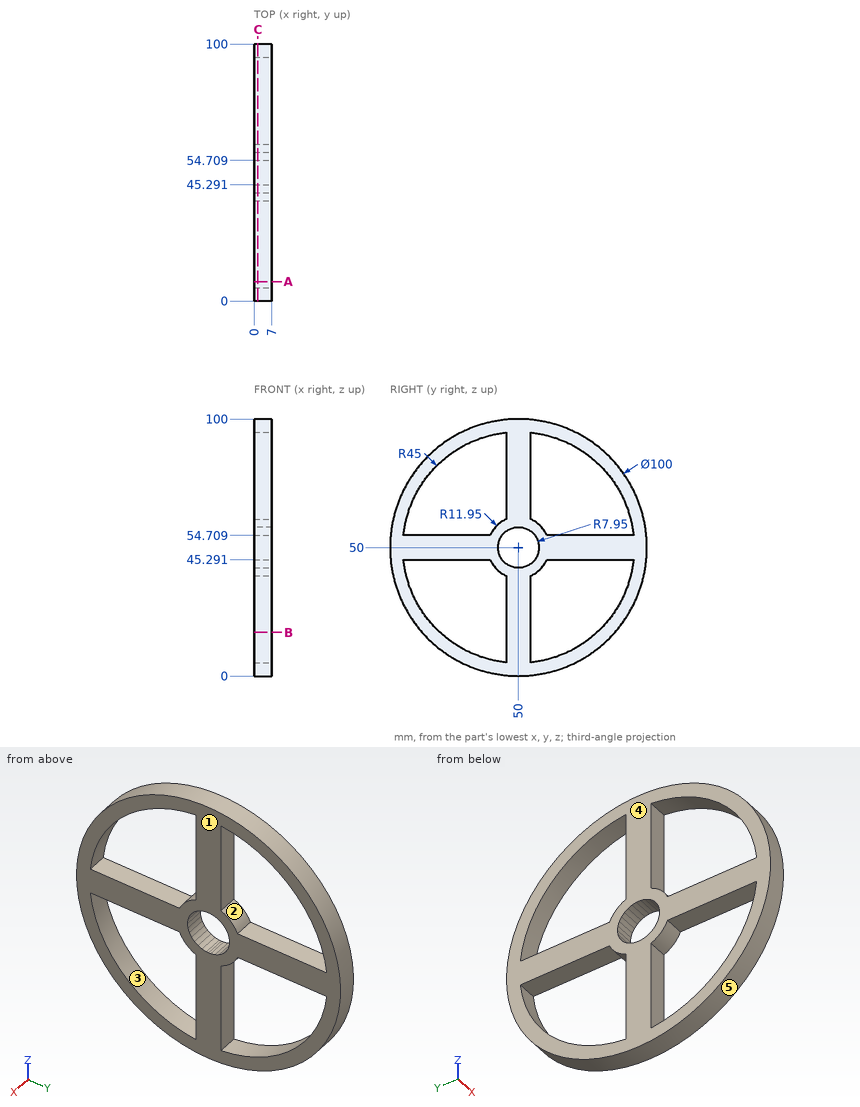
The drawing under review shows one solid part. Ordinate dimensions are in mm from its lowest x, y, z. A direction names the side the tool comes from. Coordinates: 2 decimals unless noted, no trailing zeros. Loops run counter-clockwise (first coordinate to the right, second up) from the corner with the lowest first, then second, coordinate; pieces in that order, holes last.
Item 1: Draft analysis for pull direction Y (two halves, no side actions). For the marked faces 3, 4 and 5, state which applies: pulls with the +Y half, pulls with the -Y half, needs draft (parallel to the pull), parting line crosses it, or undercut.
Completed:
face 3: undercut
face 4: needs draft
face 5: parting line crosses it
Item 2: Clearance check with flat-ended pins moving along their axes: pin 1 (2 mm diameter, centred on x = 4.5, z = 29.5, fed in from +Y); pin 2 (2 mm diameter, centred on x = 4.5, y = 79, fed in from +Z) (1 decimal); pin 3 (2 mm diameter, centred on x = 3, z = 41, fed in from -Y); pin 4 (3 mm diameter, centred on y = 82, z = 42.5, fed in from -X). State where each tip first meets the part, or that it passes through.
Completed:
pin 1: stops at y = 96.04
pin 2: stops at z = 91.4
pin 3: stops at y = 0.64
pin 4: passes through
Item 3: For the marked faces 1 and 2, list the 3-axis set-ups (+Z, -Z, +X, -X, +Y, -Y) from which the entire face can be reached by the end or side of a thin tool; tool diameter is ignored.
Completed:
face 1: +Z, -Z, +X, +Y, -Y
face 2: +X, -X
Item 4: Add section C-C (x = 1.5). Give the number of separate pieces and of enclosed holes in the cut face, and give its area (3 significant figures).
Completed:
separate pieces: 1
enclosed holes: 5
area: 3,000 mm2
Item 5: Add section B-B (z = 17). Write out the cut boundary in (x, y).
Completed:
outline: (0, 12.44) - (7, 12.44) - (7, 19.41) - (0, 19.41) - close; (0, 45.29) - (7, 45.29) - (7, 54.71) - (0, 54.71) - close; (0, 80.59) - (7, 80.59) - (7, 87.56) - (0, 87.56) - close
Item 6: Wall thickness on L1, parallel to Z at x = 5.25, y = 77; L2, parallel to Y at x = 1.75, z = 72.5; L3, parallel to Y at x = 4.5, z = 41: over which ranges is each line inside the solid? List them lowest first.
Completed:
L1: z = 7.92 to 14, 45.29 to 54.71, 86 to 92.08
L2: y = 5.35 to 11.03, 45.29 to 54.71, 88.97 to 94.65
L3: y = 0.82 to 5.91, 42.14 to 57.86, 94.09 to 99.18
Item 7: Add section A-A (y = 7.5). Write out the cut boundary in (x, z).
Completed:
outline: (0, 23.66) - (7, 23.66) - (7, 35.21) - (0, 35.21) - close; (0, 45.29) - (7, 45.29) - (7, 54.71) - (0, 54.71) - close; (0, 64.79) - (7, 64.79) - (7, 76.34) - (0, 76.34) - close
